Verification items for the finished model (mm, model axes). A direction names the side the tool comes from. Coordinates: 2 decimals unless noted, no trailing zeros. Order: outer loops, then holes, each group sorted by start corner. A loop starts at its lowest first (then second) coordinate and runs counter-clockwise, first axis right, second up. Notation, with made-up numbers: M 70,54 L 95,54 A21 cw 95,73 Z; hole C -32,-18 d7. An arc over 180 degrees is marked long. Return JSON: item names as keys, results as strings. Group by question number.
1. Set-up check for faces 1 (the flat face through (1.394, 2.374, 4.93)), 2 (the cylindrical face through (0.748, 0.976, 5.538)), 3 (the flat face through (-1.3, -1.4, 0)): record each of +Z, -Z, +X, -X, +Y, -Y from which the full face is reachable in a straight line by a thin tool's end or side.
2. Section check C-C, the plane x = 1.9. Record the cut outline in (y, z), plus the area to 3 significant figures.
3. Section check B-B, the plane z = -1.75. Record the cut outline in (x, y), plus the area to 3 significant figures.
4. Material ranges on line 1 along Y through (x, z) = (0, 2.25); line 2 along X through (y, z) = (0, 5.5); line 3 along Z through (x, y) = (0.8, 2), recorded low to high.
5. Gauge pin test, flat ends, axial feed: pin 1 (1 mm diameter, centred on x = -1.5, z = -1, fed in from +Y); pin 2 (1 mm diameter, centred on x = 0.5, y = 2.5, fed in from -Z). Record the tip position at first contact, or that the pin passes through.
6. Section check A-A, the plane z = 2.5. Record the cut outline in (x, y).
Autodesk Inventor part; units mm, degrees
ref_plane "YZ Plane" through (0, 0, 0) normal (1, 0, 0) x (0, 1, 0)
ref_plane "XZ Plane" through (0, 0, 0) normal (0, 1, 0) x (-1, 0, 0)
ref_plane "XY Plane" through (0, 0, 0) normal (0, 0, 1) x (1, 0, 0)
sketch "Sketch1" plane through (0, 0, 0) normal (0, 0, 1) x (1, 0, 0)
  line L0 (-2.75, 1.59) -> (0, 3.18)
  line L1 (0, -3.18) -> (-2.75, -1.59)
  line L2 (-2.75, 1.59) -> (-2.75, -1.59)
  line L3 (2.75, 1.59) -> (0, 3.18)
  line L4 (0, -3.18) -> (2.75, -1.59)
  line L5 (2.75, 1.59) -> (2.75, -1.59)
  point P0 (0, 0)
extrude "Extrusion1" add sketch "Sketch1" along normal blind 10
sketch "Sketch2" plane through (0, 0, 10) normal (0, 0, 1) x (1, 0, 0)
  circle A0 centre (0, 0) radius 1.5
  dimension "d20" = 3
hole "Hole1" at (0, 0, 10) direction (0, 0, -1) diameter 2.459 depth 8.8 tip angle 118
fillet "Fillet1" radius 0.1 6 edges at (0, 3.18, 5) (2.75, 1.59, 5) (-2.75, 1.59, 5) (2.75, -1.59, 5) (0, -3.18, 5) (-2.75, -1.59, 5)
sketch "Sketch4" plane through (0, 0, 0) normal (0, 0, -1) x (-1, 0, 0)
  circle A0 centre (0, 0) radius 1.5
  dimension "d29" = 3
extrude "Extrusion2" add sketch "Sketch4" along normal blind 6.4
thread "Thread1"
fillet "Fillet2" radius 0.2 1 edges at (1.5, 0, -6.4)
properties part number "spacer 10mm" material "Steel, Mild"
Answers follow:
{
 "1": {"face 1": "+Z, -Z, +X, +Y", "face 2": "+Z", "face 3": "-Z"},
 "2": {"outline": "M -2.08,0 L 2.08,0 L 2.08,10 L -2.08,10 Z", "area": "41.6 mm^2"},
 "3": {"outline": "C 0,0 d3", "area": "7.07 mm^2"},
 "4": {"line 1": "-3.16 to -1.23, 1.23 to 3.16", "line 2": "-2.75 to -1.23, 1.23 to 2.75", "line 3": "0 to 10"},
 "5": {"pin 1": "y = 1.12", "pin 2": "z = 0"},
 "6": {"outline": "M -2.75,-1.53 A0.1 ccw -2.7,-1.62 L -0.05,-3.15 A0.1 ccw 0.05,-3.15 L 2.7,-1.62 A0.1 ccw 2.75,-1.53 L 2.75,1.53 A0.1 ccw 2.7,1.62 L 0.05,3.15 A0.1 ccw -0.05,3.15 L -2.7,1.62 A0.1 ccw -2.75,1.53 Z; hole C 0,0 d2.46"}
}
